Build history of the part. All positions in model axes, mm. Face numbers are marked on the shaded views. A direction names the side the tool comes from. Give positions to 0.01 mm unless a question says otherwise; leave off trailing zeros. Order: outer loops, then holes, each group sorted by start corner. A loop starts at its lowest first (then second) coordinate and runs counter-clockwise, first axis right, second up. Notation, with made-up numbers: M 28,50.25 L 54,50.25 A23 ccw 54,80.25 Z; hole C 87,30 d8. An arc over 180 degrees is marked long. Use CSV: the item, a comma, the result in double quotes. Start each with the question number.
Item 1: Band-saw the part on A-A on z = -27.5. Write the cut outline in (x, y).
Item 2: Band-saw the part on B-B on y = 23.5. Write the cut outline in (x, z).
Item 3: Band-saw the part on C-C on y = 15. Write the cut outline in (x, z).
Item 4: Pin check, flat tips, straight feed: P1, Ø1.5, axis at y = -40.5, z = 13, coming from the +X side; P2, Ø20, axis at x = 50.5, z = -12.5, coming from the -Y side; P3, Ø2, axis at x = -32.5, z = -4, coming from the +Y side; P4, Ø6.5, axis at y = 15, z = -27.5, coming from the +X side. Stop position of each tip, or through.
Item 5: Which spindle directions (+Z, -Z, +X, -X, +Y, -Y) get a long thin tool onto all of the face, cutting with end or side? Do the marked faces 4, 5 and 6. Say none if no direction does.
Item 6: Two-plate mould, pull along X, no slides. Class the marked faces 1, 2 and 3: pulls with the +X half, pulls with the -X half, needs draft (parallel to the pull), parting line crosses it, or undercut.
Item 7: Band-saw the part on D-D on y = -25. Write the cut outline in (x, z), plus the area to 3 significant figures.
Item 8: Wall check: line 1 along Y through (x, z) = (25, 51); line 2 along X through (y, z) = (19, -52.5); line 3 along X through (y, z) = (-24, 22.5). Give the ranges that are in metal, low to high.
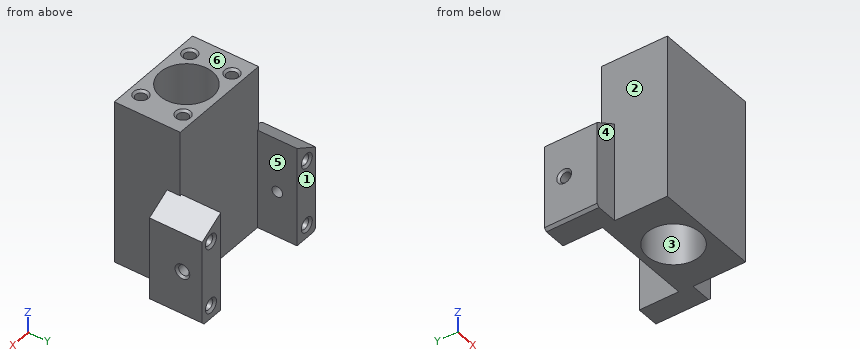
Autodesk Inventor part; units mm, degrees
ref_plane "YZ Plane" through (0, 0, 0) normal (1, 0, 0) x (0, 1, 0)
ref_plane "XZ Plane" through (0, 0, 0) normal (0, 1, 0) x (-1, 0, 0)
ref_plane "XY Plane" through (0, 0, 0) normal (0, 0, 1) x (1, 0, 0)
sketch "Эскиз1" plane through (0, 0, 0) normal (0, 1, 0) x (-1, 0, 0)
  line L0 (-40, 62.5) -> (40, 62.5)
  line L1 (40, 62.5) -> (40, -62.5)
  line L2 (40, -62.5) -> (-40, -62.5)
  line L3 (-40, -62.5) -> (-40, 62.5)
  line L4 (-40, 62.5) -> (40, -62.5) construction
  line L5 (40, 62.5) -> (-40, -62.5) construction
  line L6 (0, -62.5) -> (-58, -62.5)
  line L7 (-58, -62.5) -> (-58, 2.5)
  line L8 (-58, 2.5) -> (-39, 13.4697)
  line L9 (-58, -62.5) -> (-39, -62.5)
  line L10 (-39, -62.5) -> (-39, 13.4697)
  line L11 (0, 62.5) -> (0, -62.5)
  line L12 (0, -62.5) -> (58, -62.5)
  line L13 (58, -62.5) -> (58, 2.5)
  line L14 (58, 2.5) -> (39, 13.4697)
  line L15 (39, -62.5) -> (39, 13.4697)
  point P0 (0, 0)
  point P1 (-40, 12.8923)
  point P2 (40, 12.8923)
  dimension "d0" = 80
  dimension "d1" = 125
  dimension "d2" = 58
  dimension "d3" = 65
  dimension "d4" = 120
  dimension "d5" = 19
extrude "Выдавливание1" add sketch "Эскиз1" along normal blind 30 and the other way blind 10 contours L8 L10 L2 L3 | L3 L6 L7 L8 | L14 L13 L12 L1 | L1 L2 L15 L14
extrude "Выдавливание2" add sketch "Эскиз1" against normal blind 50 contours L0 L11 L2 L10 L8 L3 | L0 L1 L14 L15 L2 L11 | L8 L10 L2 L3 | L1 L2 L15 L14
sketch "Эскиз3" plane through (0, 30, 0) normal (0, 1, 0) x (1, 0, 0)
  line L0 (39, 62.5) -> (-39, 62.5)
  line L1 (0, 62.5) -> (49, 62.5)
  line L2 (49, 62.5) -> (49, 52.5)
  line L3 (49, 52.5) -> (49, 2.5)
  point P0 (0, 0)
  point P1 (40, 62.5)
  point P2 (-40, 62.5)
  dimension "d15" = 49
  dimension "d16" = 10
  dimension "d17" = 50
hole "Отверстие1" at (49, 30, -2.5) at (49, 30, -52.5) direction (0, -1, 0) diameter 8 depth 18 tip angle 118
thread "Резьба1"
thread "Резьба2"
sketch "Эскиз4" plane through (0, 30, 0) normal (0, 1, 0) x (1, 0, 0)
  line L0 (39, 62.5) -> (-39, 62.5)
  line L1 (0, 62.5) -> (-49, 62.5)
  line L2 (-49, 62.5) -> (-49, 52.5)
  line L3 (-49, 52.5) -> (-49, 2.5)
  point P0 (0, 0)
  dimension "d29" = 49
  dimension "d30" = 10
  dimension "d31" = 50
hole "Отверстие2" at (-49, 30, -52.5) at (-49, 30, -2.5) direction (0, -1, 0) diameter 8 depth 18 tip angle 118
thread "Резьба3"
thread "Резьба4"
sketch "Эскиз5" plane through (-40, 0, 62.5) normal (0, 0, 1) x (1, 0, 0)
  line L0 (40, 0) -> (40, -50)
  line L1 (0, -50) -> (80, -50)
  line L2 (0, -10) -> (0, -50)
  line L3 (0, -25) -> (80, -25)
  line L4 (80, -10) -> (80, -50)
  line L5 (15, -41) -> (65, -41)
  line L6 (65, -41) -> (65, -9)
  line L7 (65, -9) -> (15, -9)
  line L8 (15, -9) -> (15, -41)
  line L9 (15, -41) -> (65, -9) construction
  line L10 (65, -41) -> (15, -9) construction
  point P0 (40, -25)
  dimension "d44" = 50
  dimension "d45" = 32
hole "Отверстие3" at (0, -25, 62.5) direction (0, 0, -1) diameter 40 end through all
hole "Отверстие4" at (25, -41, 62.5) at (-25, -41, 62.5) at (-25, -9, 62.5) at (25, -9, 62.5) direction (0, 0, -1) diameter 8 depth 18 tip angle 118
thread "Резьба5"
thread "Резьба6"
thread "Резьба7"
thread "Резьба8"
sketch "Эскиз6" plane through (58, -10, -62.5) normal (1, 0, 0) x (0, 0, -1)
  line L0 (0, 10) -> (0, 40)
  line L1 (0, 10) -> (0, 25)
  line L2 (0, 25) -> (-35, 25)
  point P0 (-62.5, 10)
  dimension "d69" = 15
  dimension "d70" = 35
hole "Отверстие5" at (58, 15, -27.5) direction (-1, 0, 0) diameter 8 depth 116
chamfer "Фаска1" distance 1.6 angle 45 1 edges at (-58, 15, -23.5)
chamfer "Фаска2" distance 1.6 angle 45 1 edges at (58, 15, -23.5)
chamfer "Фаска3" distance 1.6 angle 45 4 edges at (-25, -37, 62.5) (25, -37, 62.5) (-25, -5, 62.5) (25, -5, 62.5)
thread "Резьба9"
chamfer "Фаска4" distance 1.6 angle 45 4 edges at (49, 30, -56.5) (49, 30, -6.5) (-49, 30, -56.5) (-49, 30, -6.5)
chamfer "Фаска5" distance 2 angle 45 2 edges at (58, 10, -62.5) (-58, 10, -62.5)
properties part number "Губка-2"
Model answer:
1,outline,"M -58,-10 L -40,-10 L -40,-50 L 40,-50 L 40,-10 L 58,-10 L 58,9.4 L 56.4,11 L 39,11 L 39,0 L -39,0 L -39,11 L -56.4,11 L -58,9.4 Z; M -58,20.6 L -56.4,19 L -39,19 L -39,30 L -58,30 Z; M 39,19 L 56.4,19 L 58,20.6 L 58,30 L 39,30 Z; hole C 0,-25 d40"
2,outline,"M -58,-60.5 L -56,-62.5 L -39,-62.5 L -39,13.47 L -58,2.5 Z; M 39,-62.5 L 56,-62.5 L 58,-60.5 L 58,2.5 L 39,13.47 Z; hole C -49,-52.5 d8; hole C -49,-2.5 d8; hole C 49,-52.5 d8; hole C 49,-2.5 d8"
3,outline,"M -58,-60.5 L -56,-62.5 L -39,-62.5 L -39,-31.5 L -56.4,-31.5 L -58,-33.1 Z; M -58,-21.9 L -56.4,-23.5 L -39,-23.5 L -39,13.47 L -58,2.5 Z; M 39,-62.5 L 56,-62.5 L 58,-60.5 L 58,-33.1 L 56.4,-31.5 L 39,-31.5 Z; M 39,-23.5 L 56.4,-23.5 L 58,-21.9 L 58,2.5 L 39,13.47 Z; hole C -49,-52.5 d8; hole C -49,-2.5 d8; hole C 49,-52.5 d8; hole C 49,-2.5 d8"
4,P1,"stops at x = 40"
4,P2,"stops at y = -10"
4,P3,"stops at y = 0"
4,P4,"passes through"
5,face 4,"+Z, -Z, -X, -Y"
5,face 5,"+Z, -Z, +Y"
5,face 6,"+Z, +X, -X, +Y, -Y"
6,face 1,"needs draft"
6,face 2,"pulls with the -X half"
6,face 3,"undercut"
7,outline,"M -40,-62.5 L -20,-62.5 L -20,62.5 L -40,62.5 Z; M 20,-62.5 L 40,-62.5 L 40,62.5 L 20,62.5 Z"
7,area,"5,000 mm^2"
8,line 1,"y = -50 to -45, -37 to -13, -5 to 0"
8,line 2,"x = -58 to -53, -45 to -39, 39 to 45, 53 to 58"
8,line 3,"x = -40 to -19.97, 19.97 to 40"
